Here's how the part is built. I have some questions about the finished solid (model axes, mm). A direction names the side the tool comes from. Coordinates: 2 decimals unless noted, no trailing zeros. Loops run counter-clockwise (first coordinate to the right, second up) from the corner with the lowest first, then second, coordinate; pieces in that order, holes last. Notation, with made-up numbers: (40.25, -3) - (74.25, -3) arc R29 cw to (74.25, 28) - close; hole circle Ø8 at (12.25, 60). An arc over 180 degrees is marked (long way). Use a Markdown table: item, result.
```python
from build123d import *

# Parameters (mm, degrees)
SKETCH1_W                = 50.8
SKETCH1_H                = 50.8
BOSS_EXTRUDE1_DEPTH      = 2
SKETCH2_R                = 15
SKETCH2_R_2              = 13
BOSS_EXTRUDE2_DEPTH      = 20
CHAMFER1_SIZE            = 1
FILLET1_R                = 5
BOSS_EXTRUDE4_DEPTH      = 1
BOSS_EXTRUDE4_DEPTH_BACK = 1
BOSS_EXTRUDE5_DEPTH      = 1
BOSS_EXTRUDE5_DEPTH_BACK = 1
SKETCH7_R                = 6.35
CUT_EXTRUDE1_DEPTH       = 11
CHAMFER2_SIZE            = 3


with BuildPart() as part:
    # Sketch1 → Boss-Extrude1 (new body)
    with BuildSketch(Plane(origin=(0, 0, 0), x_dir=(1, 0, 0), z_dir=(0, 1, 0))):
        Rectangle(SKETCH1_W, SKETCH1_H)
    extrude(amount=BOSS_EXTRUDE1_DEPTH)

    # Sketch2 → Boss-Extrude2 (add)
    with BuildSketch(Plane(origin=(0, 2, 0), x_dir=(1, 0, 0), z_dir=(0, 1, 0))):
        with Locations(Location((0, 0, 0), (0, 0, 270))):
            Circle(SKETCH2_R)
        with Locations(Location((0, 0, 0), (0, 0, 270))):
            Circle(SKETCH2_R_2, mode=Mode.SUBTRACT)
    extrude(amount=BOSS_EXTRUDE2_DEPTH)

    # Chamfer1
    chamfer1_edges = [part.edges().sort_by_distance(p)[0] for p in [
        (0, 22, -15),
    ]]
    chamfer(chamfer1_edges, length=CHAMFER1_SIZE)

    # Fillet1
    fillet1_edges = [part.edges().sort_by_distance(p)[0] for p in [
        (25.4, 1, 25.4),
        (-25.4, 1, 25.4),
        (-25.4, 1, -25.4),
        (25.4, 1, -25.4),
    ]]
    fillet(fillet1_edges, radius=FILLET1_R)

    # Sketch5 → Boss-Extrude4 (add, two sides: drawn at the far end of the back side and taken through both)
    with BuildSketch(Plane(origin=(0, 0, 0), x_dir=(-0.7071067811865476, 0, -0.7071067811865476), z_dir=(0.7071067811865476, 0, -0.7071067811865476)).offset(-BOSS_EXTRUDE4_DEPTH_BACK)):
        Polygon((-15, 21), (-28.849956672, 2), (-14.211911486, 2), (-14.211911486, 20.928757868), align=None)
        Polygon((15, 21), (28.849956672, 2), (14.236311105, 2), (14.236311105, 20.928757868), align=None)
    extrude(amount=BOSS_EXTRUDE4_DEPTH + BOSS_EXTRUDE4_DEPTH_BACK)

    # Sketch6 → Boss-Extrude5 (add, two sides: drawn at the far end of the back side and taken through both)
    with BuildSketch(Plane(origin=(0, 0, 0), x_dir=(0.7071067811865475, 0, -0.7071067811865476), z_dir=(0.7071067811865476, 0, 0.7071067811865475)).offset(-BOSS_EXTRUDE5_DEPTH_BACK)):
        Polygon((-15, 21), (-28.849956672, 2), (-14.171301729, 2), (-14.171301729, 20.395924466), align=None)
        Polygon((15, 21), (28.849956672, 2), (14.152219343, 2), (14.152219343, 20.382014455), align=None)
    extrude(amount=BOSS_EXTRUDE5_DEPTH + BOSS_EXTRUDE5_DEPTH_BACK)

    # Sketch7 → Cut-Extrude1 (cut)
    with BuildSketch(Plane(origin=(0, 2, 0), x_dir=(1, 0, 0), z_dir=(0, 1, 0))):
        with Locations(Location((-0.199881489, -0.225905454, 0), (0, 0, 270))):
            Circle(SKETCH7_R)
    extrude(amount=-CUT_EXTRUDE1_DEPTH, mode=Mode.SUBTRACT)

    # Chamfer2
    chamfer2_edges = [part.edges().sort_by_distance(p)[0] for p in [
        (0, 2, -15),
        (15, 2, 0),
        (-15, 2, 0),
        (0, 2, 15),
    ]]
    chamfer(chamfer2_edges, length=CHAMFER2_SIZE)


solid = part.part
```
Q1. Will these pins go through, and if not, where does the flat tip stop? P1, Ø8, axis at x = 5.5, z = -2, coming from the +Y side; P2, Ø5, axis at y = 10.5, z = 1, coming from the -X side; P3, Ø4, axis at y = 11, z = -16, coming from the +X side; P4, Ø1, axis at x = -15.5, z = -19.5, coming from the -Y side.
Check values:
| item | result |
|---|---|
| P1 | y = 2 |
| P2 | x = -15 |
| P3 | x = 17.5 |
| P4 | y = 0 |
Q2. If we mould it in two halves opening along X, with no side actions, what happens to faces 1 (the face through (0, 13, 15)), 2 (the face through (6, 2, -3)), 3 (the face through (-9.3, 22, 9.3)), 4 (the face through (-15.445, 11.633, 15.425))? For each: pulls with the +X half, pulls with the -X half, needs draft (parallel to the pull), parting line crosses it, or undercut.
Check values:
| item | result |
|---|---|
| face 1 | undercut |
| face 2 | undercut |
| face 3 | needs draft |
| face 4 | pulls with the -X half |
Q3. I want a section at A-A, the plane y = 17.75. Write out the boundary of the cut face in (x, z).
Check values:
| item | result |
|---|---|
| outline | (-12.99, -11.57) - (-11.57, -12.99) - (-9.88, -11.29) arc R15 ccw to (9.88, -11.29) - (11.57, -12.99) - (12.99, -11.57) - (11.29, -9.88) arc R15 ccw to (11.29, 9.88) - (12.99, 11.57) - (11.57, 12.99) - (9.88, 11.29) arc R15 ccw to (-9.88, 11.29) - (-11.57, 12.99) - (-12.99, 11.57) - (-11.29, 9.88) arc R15 ccw to (-11.29, -9.88) - close; hole circle Ø26 at (0, 0) |
Q4. I want a section at B-B, the plane z = 0. Write out the boundary of the cut face in (x, y).
Check values:
| item | result |
|---|---|
| outline | (-25.4, 0) - (-6.55, 0) - (-6.55, 2) - (-13, 2) - (-13, 22) - (-14, 22) - (-15, 21) - (-15, 5) - (-18, 2) - (-25.4, 2) - close; (6.15, 0) - (25.4, 0) - (25.4, 2) - (18, 2) - (15, 5) - (15, 21) - (14, 22) - (13, 22) - (13, 2) - (6.15, 2) - close |
Q5. I want a section at D-D, the plane y = 10.5. Write out the boundary of the cut face in (x, z), then the cut area to 3 significant figures.
Check values:
| item | result |
|---|---|
| outline | (-16.73, -15.31) - (-15.31, -16.73) - (-9.88, -11.29) arc R15 ccw to (9.88, -11.29) - (15.31, -16.73) - (16.73, -15.31) - (11.29, -9.88) arc R15 ccw to (11.29, 9.88) - (16.73, 15.31) - (15.31, 16.73) - (9.88, 11.29) arc R15 ccw to (-9.88, 11.29) - (-15.31, 16.73) - (-16.73, 15.31) - (-11.29, 9.88) arc R15 ccw to (-11.29, -9.88) - close; hole circle Ø26 at (0, 0) |
| area | 237 mm^2 |
Q6. Which directions (+Z, -Z, +X, -X, +Y, -Y) give clear straight access to the entire face, cutting with the end or side of a thin tool? Please do faces 5 (the face through (14.086, 7.411, -12.672)), 6 (the face through (-12.672, 7.411, 14.086)), 7 (the face through (12.672, 7.411, -14.086)), 8 (the face through (-6, 2, -17.3)).
Check values:
| item | result |
|---|---|
| face 5 | +X, +Y |
| face 6 | +Z, +Y |
| face 7 | -Z, +Y |
| face 8 | +Y |
Q7. Please list where these lines run through material, in increasing order: L1, parallel to X at y = 16.5, z = -0.5; L2, parallel to Y at x = 18.5, z = 20; L3, parallel to X at y = 3, z = -14. Write a range as from..to.
Check values:
| item | result |
|---|---|
| L1 | -14.99..-12.99, 12.99..14.99 |
| L2 | 0..2 |
| L3 | -15.41..-12.59, -9.64..9.64, 12.59..15.41 |
Q8. I want a section at C-C, the plane z = 19. Write out the boundary of the cut face in (x, y).
Check values:
| item | result |
|---|---|
| outline | (-25.4, 0) - (25.4, 0) - (25.4, 2) - (20.41, 2) - (20.41, 3.34) - (17.59, 6.09) - (17.59, 2) - (-17.59, 2) - (-17.59, 6.09) - (-20.41, 3.34) - (-20.41, 2) - (-25.4, 2) - close |
